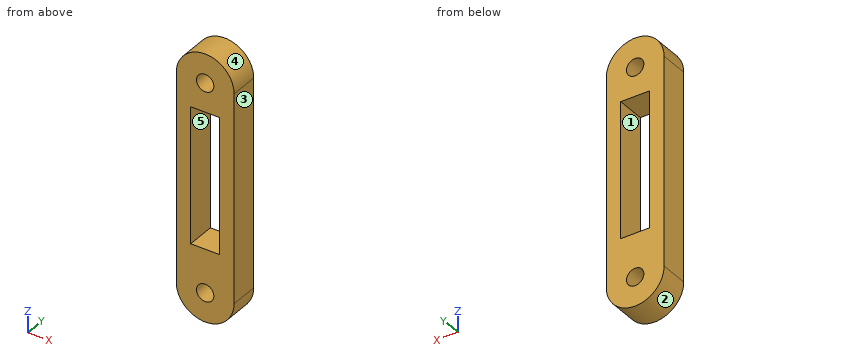
```python
from build123d import *

# Parameters (mm, degrees)
EXTRUDE_1_DEPTH     = 5
SKETCH_3_W          = 5
SKETCH_3_H          = 23.5
CUT_EXTRUDE_1_DEPTH = 5
SKETCH_4_R          = 1.5
CUT_EXTRUDE_2_DEPTH = 5


with BuildPart() as part:
    # 草图2 → 凸台-拉伸1 (new body)
    with BuildSketch(Plane(origin=(0, 0, 0), x_dir=(1, 0, 0), z_dir=(0, 1, 0))):
        with BuildLine():
            Line((5, 18), (5, -18))
            ThreePointArc((5, -18), (0, -23), (-5, -18))
            Line((-5, -18), (-5, 18))
            ThreePointArc((-5, 18), (0, 23), (5, 18))
        make_face()
    extrude(amount=EXTRUDE_1_DEPTH)

    # 草图3 → 切除-拉伸1 (cut)
    with BuildSketch(Plane.XZ):
        with Locations((0, 1.25)):
            Rectangle(SKETCH_3_W, SKETCH_3_H)
    extrude(amount=-CUT_EXTRUDE_1_DEPTH, mode=Mode.SUBTRACT)

    # 草图4 → 切除-拉伸2 (cut)
    with BuildSketch(Plane.XZ):
        with Locations(Location((0, 18, 0), (0, 0, 270))):
            Circle(SKETCH_4_R)
        with Locations(Location((0, -18, 0), (0, 0, 90))):
            Circle(SKETCH_4_R)
    extrude(amount=-CUT_EXTRUDE_2_DEPTH, mode=Mode.SUBTRACT)


solid = part.part
```
Geometry check sheet. Reference: the model listing, model coordinates, mm. Face numbers are marked on the shaded views. A direction names the side the tool comes from. Give positions to 0.01 mm unless a question says otherwise; leave off trailing zeros. Loops run counter-clockwise (first coordinate to the right, second up) from the corner with the lowest first, then second, coordinate; pieces in that order, holes last. Notation, with made-up numbers: M 72,33.25 L 126,33.25 A19 cw 126,37.25 Z; hole C 5.5,-30 d11. An arc over 180 degrees is marked long. Write item = value, one per line.
(1) Sectioned sample at D-D, the plane z = 17. Record the cut outline in (x, y), plus the area to 3 significant figures.
Answer below:
outline = M -5,0 L -1.12,0 L -1.12,5 L -5,5 Z; M 1.12,0 L 5,0 L 5,5 L 1.12,5 Z
area = 38.8 mm2
(2) Tool access check on the marked faces 1 and 2. Record the directions out of +Z, -Z, +X, -X, +Y, -Y that give a thin tool (end or side, any length) a straight path to the whole face; none if there is none.
Answer below:
face_1 = +Y, -Y
face_2 = -Z, +Y, -Y
(3) Sectioned sample at C-C, the plane z = 2. Record the cut outline in (x, y).
Answer below:
outline = M -5,0 L -2.5,0 L -2.5,5 L -5,5 Z; M 2.5,0 L 5,0 L 5,5 L 2.5,5 Z
(4) Gauge pin test, flat end, axial feed: pin 1 Ø2 at (x, y) = (3, 1.5) entering from +Z. Record the tip position at first contact, or that the pin passes through.
Answer below:
pin_1 = 22.58
(5) Release check for a two-part mould opening along Z. For the marked faces 3, 4 and 5 record: released by +Z, released by -Z, zero draft, split by the parting line, or undercut.
Answer below:
face_3 = zero draft
face_4 = released by +Z
face_5 = undercut
(6) Sectioned sample at B-B, the plane x = 0. Record the cut outline in (y, z).
Answer below:
outline = M 0,-23 L 5,-23 L 5,-19.5 L 0,-19.5 Z; M 0,-16.5 L 5,-16.5 L 5,-10.5 L 0,-10.5 Z; M 0,13 L 5,13 L 5,16.5 L 0,16.5 Z; M 0,19.5 L 5,19.5 L 5,23 L 0,23 Z
(7) Material ranges on line 1 (X direction, y = 1.85, z = 0.5); line 2 (X direction, y = 2.6, z = 18); line 3 (Z direction, x = 1, y = 0.9), recorded low to high. Write a range as [from, to].
Answer below:
line_1 = [-5, -2.5], [2.5, 5]
line_2 = [-5, -1.5], [1.5, 5]
line_3 = [-22.9, -19.12], [-16.88, -10.5], [13, 16.88], [19.12, 22.9]
(8) Sectioned sample at A-A, the plane y = 2.55. Record the cut outline in (x, z).
Answer below:
outline = M -5,-18 A5 ccw 5,-18 L 5,18 A5 ccw -5,18 Z; hole M -2.5,-10.5 L 2.5,-10.5 L 2.5,13 L -2.5,13 Z; hole C 0,-18 d3; hole C 0,18 d3
